Source: CAD feature listing. Evaluate the final solid. Frame: model axes, mm. A direction names the side the tool comes from. Coordinates: 2 decimals unless noted, no trailing zeros. Write each loop counter-clockwise with the first axis right and the second up, starting at its lowest first coordinate (ties: lowest second). Pieces come first, ordered by that corner, then holes. Notation, with made-up numbers: M 77,20 L 110,20 A11 ccw 110,38 Z; hole C 67,39 d6. An arc over 180 degrees is marked long. Answer as CSV lines item,"result". Start each with the question number.
1. Contact query for flat-ended pins moving along their axis: pin 1 Ø2 at (x, z) = (15.5, -4.5) entering from -Y; pin 2 Ø5 at (x, z) = (19.5, 1.5) entering from +Y; pin 3 Ø6 at (y, z) = (-2.5, -4) entering from +X; pin 4 Ø5 at (x, y) = (24.5, 2) entering from -Z. Output: stop coordinate, or through.
2. Line query: probe 1 along X at (y, z) = (4, 0.5); probe 2 along X at (y, z) = (-0.5, -3.75); probe 3 along Y at (x, z) = (16.5, -0.25). Output: solid intervals per line, ascending. Write a range as [from, to].
3. Section B-B on z = 0. Return the cut outline in (x, y).
4. Mould query, pull axis Y, two halves, no side actions, for faces 4 (the face through (35, 0, 0)), 5 (the face through (1, 1, 0)), 6 (the face through (1, -1, 0)), 7 (the face through (20.21, -0.867, -3.905)). Classes: pulls with the +Y half, pulls with the -Y half, needs draft (parallel to the pull), parting line crosses it, or undercut.
5. Reachability of faces 1 (the face through (5, 3, 3)), 2 (the face through (2, 0, 0)), 3 (the face through (0, 3, 0)) from +Z, -Z, +X, -X, +Y, -Y: full face, straight path, thin tool, end or side. Return the list, or none.
6. Section A-A on y = 0. Return the cut outline in (x, z).
7. Section C-C on x = 26.5. Return the cut outline in (y, z).
```python
from build123d import *

# Parameters (mm, degrees)
SKETCH2_W  = 13
SKETCH2_H  = 2
SLOT_DEPTH = 2


with BuildPart() as part:
    # Fillet2: read off the stored shape, not the designer's step
    # Fillet2 outline → Fillet2 (revolve)
    with BuildSketch(Plane.YX):
        with BuildLine():
            Line((4, 5), (4, 35))
            Line((4, 35), (0, 35))
            Line((0, 35), (0, 0))
            Line((0, 0), (5.696024213, 0))
            ThreePointArc((5.696024213, 0), (5.966260296, 0.105089065), (6.094502092, 0.365137703))
            Line((6.094502092, 0.365137703), (6.5, 5))
            Line((6.5, 5), (4, 5))
        make_face()
    revolve(axis=Axis((0, 0, 0), (1, 0, 0)))

    # Sketch2 → Slot (cut)
    with BuildSketch(Plane(origin=(0, 0, 0), x_dir=(0, 0, -1), z_dir=(1, 0, 0))):
        Rectangle(SKETCH2_W, SKETCH2_H)
    extrude(amount=SLOT_DEPTH, mode=Mode.SUBTRACT)


solid = part.part
```
Values:
1,pin 1,"y = -1.94"
1,pin 2,"y = 4"
1,pin 3,"x = 35"
1,pin 4,"z = -4"
2,probe 1,"[0, 5]"
2,probe 2,"[2, 35]"
2,probe 3,"[-3.99, 3.99]"
3,outline,"M 0,-5.7 A0.4 ccw 0.37,-6.09 L 5,-6.5 L 5,-4 L 35,-4 L 35,4 L 5,4 L 5,6.5 L 0.37,6.09 A0.4 ccw 0,5.7 L 0,1 L 2,1 L 2,-1 L 0,-1 Z"
4,face 4,"needs draft"
4,face 5,"undercut"
4,face 6,"undercut"
4,face 7,"parting line crosses it"
5,face 1,"+X"
5,face 2,"+Z, -Z, -X"
5,face 3,"+Z, -Z, -X, +Y, -Y"
6,outline,"M 2,-6.24 L 5,-6.5 L 5,-4 L 35,-4 L 35,4 L 5,4 L 5,6.5 L 2,6.24 Z"
7,outline,"C 0,0 d8"
